Part model, mm, in its own coordinate system. Face numbers are marked on the shaded views. A direction names the side the tool comes from. Round coordinates to 2 decimals unless told otherwise and drop trailing zeros. Loops run counter-clockwise (first coordinate to the right, second up) from the corner with the lowest first, then second, coordinate; pieces in that order, holes last. Notation, with made-up numbers: M 77.25,-36 L 110.25,-36 A18 ccw 110.25,-11 Z; hole C 83.25,11 d3. An arc over 180 degrees is marked long. Answer as CSV lines item,"result". Start each with the question number.
Item 1: Band-saw the part on B-B (z = 0). Give the cut face in (x, y), and give its area (3 significant figures).
Item 2: Mould opens along Z. For the marked faces 1, 2 and 3 say: pulls with the +Z half, pulls with the -Z half, needs draft (parallel to the pull), parting line crosses it, or undercut.
Item 3: Band-saw the part on C-C (y = 20). Give the cut face in (x, z).
Item 4: Which spindle directions (+Z, -Z, +X, -X, +Y, -Y) get a long thin tool onto all of the face, cutting with end or side? Do the marked faces 4, 5, 6, 7 and 8. Say none if no direction does.
Item 5: Wall check: line 1 (Z direction, x = 34.5, y = 11.5); line 2 (Y direction, x = 6.5, z = 44.5). Give the ranges that are in metal, low to high.
Item 6: Band-saw the part on D-D (x = -39). Give the cut face in (y, z).
Item 7: Drop flat-ended pins along their axis: pin 1 Ø4 at (x, z) = (15.5, -36) entering from +Y; pin 2 Ø1.5 at (y, z) = (23.5, 7) entering from +X; pin 3 Ø3 at (y, z) = (25.5, -25) entering from +X. Give the stop position or say it passes through.
Item 8: Band-saw the part on A-A (x = 0). Give the cut face in (y, z), and give its area (3 significant figures).
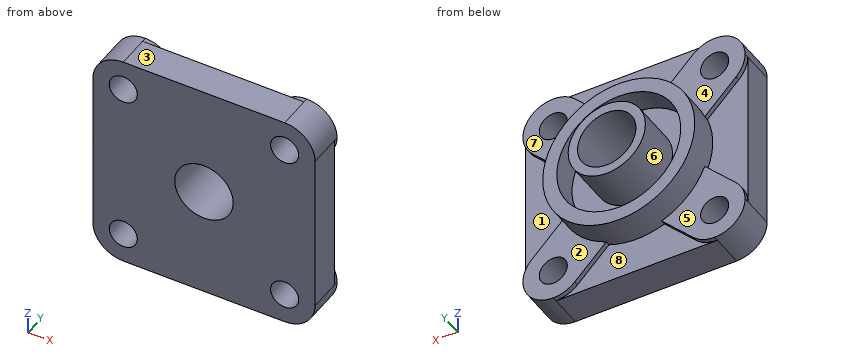
```python
from build123d import *

# Parameters (mm, degrees)
SKETCH1_W           = 95
SKETCH1_H           = 95
BOSS_EXTRUDE1_DEPTH = 14
BOSS_EXTRUDE2_DEPTH = 16
SKETCH4_R           = 32.5
BOSS_EXTRUDE3_DEPTH = 13
SKETCH5_R           = 12.5
CUT_EXTRUDE1_DEPTH  = 73.398204398
SKETCH6_R           = 26.5
SKETCH6_R_2         = 16.5
CUT_EXTRUDE2_DEPTH  = 11
BOSS_EXTRUDE4_START = 35.7
SKETCH7_R           = 16.5
SKETCH7_R_2         = 12.5
BOSS_EXTRUDE4_DEPTH = 35.7
CUT_EXTRUDE3_DEPTH  = 77.072268272
SKETCH9_R           = 6
CUT_EXTRUDE5_DEPTH  = 77.072268272


with BuildPart() as part:
    # Sketch1 → Boss-Extrude1 (new body)
    with BuildSketch(Plane(origin=(0, 0, 0), x_dir=(1, 0, 0), z_dir=(0, 1, 0))):
        Rectangle(SKETCH1_W, SKETCH1_H)
    extrude(amount=BOSS_EXTRUDE1_DEPTH)

    # Sketch2 → Boss-Extrude2 (add)
    with BuildSketch(Plane(origin=(0, 0, 0), x_dir=(1, 0, 0), z_dir=(0, 1, 0))):
        with BuildLine():
            Line((-30.254795425, 11.870019114), (-43.692388155, 25.307611845))
            ThreePointArc((-43.692388155, 25.307611845), (-43.692388155, 43.692388155), (-25.307611845, 43.692388155))
            Line((-25.307611845, 43.692388155), (-11.870019114, 30.254795425))
            ThreePointArc((-11.870019114, 30.254795425), (-22.980970389, 22.980970389), (-30.254795425, 11.870019114))
        make_face()
        with BuildLine():
            Line((11.870019114, 30.254795425), (25.307611845, 43.692388155))
            ThreePointArc((25.307611845, 43.692388155), (43.692388155, 43.692388155), (43.692388155, 25.307611845))
            Line((43.692388155, 25.307611845), (30.254795425, 11.870019114))
            ThreePointArc((30.254795425, 11.870019114), (22.980970389, 22.980970389), (11.870019114, 30.254795425))
        make_face()
        with BuildLine():
            Line((30.254795425, -11.870019114), (43.692388155, -25.307611845))
            ThreePointArc((43.692388155, -25.307611845), (43.692388155, -43.692388155), (25.307611845, -43.692388155))
            Line((25.307611845, -43.692388155), (11.870019114, -30.254795425))
            ThreePointArc((11.870019114, -30.254795425), (22.980970389, -22.980970389), (30.254795425, -11.870019114))
        make_face()
        with BuildLine():
            Line((-11.870019114, -30.254795425), (-25.307611845, -43.692388155))
            ThreePointArc((-25.307611845, -43.692388155), (-43.692388155, -43.692388155), (-43.692388155, -25.307611845))
            Line((-43.692388155, -25.307611845), (-30.254795425, -11.870019114))
            ThreePointArc((-30.254795425, -11.870019114), (-22.980970389, -22.980970389), (-11.870019114, -30.254795425))
        make_face()
    extrude(amount=BOSS_EXTRUDE2_DEPTH)

    # Sketch4 → Boss-Extrude3 (add)
    with BuildSketch(Plane(origin=(0, 14, 0), x_dir=(1, 0, 0), z_dir=(0, 1, 0))):
        with Locations(Location((0, 0, 0), (0, 0, 111.421821522))):
            Circle(SKETCH4_R)
    extrude(amount=BOSS_EXTRUDE3_DEPTH)

    # Sketch5 → Cut-Extrude1 (cut, through all)
    with BuildSketch(Plane(origin=(0, 27, 0), x_dir=(1, 0, 0), z_dir=(0, 1, 0))):
        with Locations(Location((0, 0, 0), (0, 0, 270))):
            Circle(SKETCH5_R)
    extrude(amount=-CUT_EXTRUDE1_DEPTH, mode=Mode.SUBTRACT)

    # Sketch6 → Cut-Extrude2 (cut)
    with BuildSketch(Plane(origin=(0, 27, 0), x_dir=(1, 0, 0), z_dir=(0, 1, 0))):
        with Locations(Location((0, 0, 0), (0, 0, 270))):
            Circle(SKETCH6_R)
        with Locations(Location((0, 0, 0), (0, 0, 270))):
            Circle(SKETCH6_R_2, mode=Mode.SUBTRACT)
    extrude(amount=-CUT_EXTRUDE2_DEPTH, mode=Mode.SUBTRACT)

    # Sketch7 → Boss-Extrude4 (add)
    with BuildSketch(Plane(origin=(0, 0, 0), x_dir=(1, 0, 0), z_dir=(0, 1, 0)).offset(BOSS_EXTRUDE4_START)):
        with Locations(Location((0, 0, 0), (0, 0, 270))):
            Circle(SKETCH7_R)
        with Locations(Location((0, 0, 0), (0, 0, 270))):
            Circle(SKETCH7_R_2, mode=Mode.SUBTRACT)
    extrude(amount=-BOSS_EXTRUDE4_DEPTH)

    # Sketch8 → Cut-Extrude3 (cut, through all)
    with BuildSketch(Plane(origin=(0, 0, 0), x_dir=(1, 0, 0), z_dir=(0, 1, 0))):
        with BuildLine():
            Line((-47.5, -34.5), (-47.5, -47.5))
            Line((-47.5, -47.5), (-34.5, -47.5))
            ThreePointArc((-34.5, -47.5), (-43.692388155, -43.692388155), (-47.5, -34.5))
        make_face()
        with BuildLine():
            Line((-34.5, 47.5), (-47.5, 47.5))
            Line((-47.5, 47.5), (-47.5, 34.5))
            ThreePointArc((-47.5, 34.5), (-43.692388155, 43.692388155), (-34.5, 47.5))
        make_face()
        with BuildLine():
            Line((47.5, 34.5), (47.5, 47.5))
            Line((47.5, 47.5), (34.5, 47.5))
            ThreePointArc((34.5, 47.5), (43.692388155, 43.692388155), (47.5, 34.5))
        make_face()
        with BuildLine():
            Line((34.5, -47.5), (47.5, -47.5))
            Line((47.5, -47.5), (47.5, -34.5))
            ThreePointArc((47.5, -34.5), (43.692388155, -43.692388155), (34.5, -47.5))
        make_face()
    extrude(amount=CUT_EXTRUDE3_DEPTH, mode=Mode.SUBTRACT)

    # Sketch9 → Cut-Extrude5 (cut, through all)
    with BuildSketch(Plane(origin=(0, 0, 0), x_dir=(1, 0, 0), z_dir=(0, 1, 0))):
        with Locations(Location((-34.5, 34.5, 0), (0, 0, 90))):
            Circle(SKETCH9_R)
        with Locations(Location((34.5, 34.5, 0), (0, 0, 90))):
            Circle(SKETCH9_R)
        with Locations(Location((34.5, -34.5, 0), (0, 0, 90))):
            Circle(SKETCH9_R)
        with Locations(Location((-34.5, -34.5, 0), (0, 0, 90))):
            Circle(SKETCH9_R)
    extrude(amount=CUT_EXTRUDE5_DEPTH, mode=Mode.SUBTRACT)


solid = part.part
```
Answer block:
1,outline,"M -47.5,0 L -12.5,0 L -12.5,35.7 L -16.5,35.7 L -16.5,16 L -26.5,16 L -26.5,27 L -32.5,27 L -32.5,14 L -47.5,14 Z; M 12.5,0 L 47.5,0 L 47.5,14 L 32.5,14 L 32.5,27 L 26.5,27 L 26.5,16 L 16.5,16 L 16.5,35.7 L 12.5,35.7 Z"
1,area,"1,350 mm^2"
2,face 1,"undercut"
2,face 2,"needs draft"
2,face 3,"pulls with the +Z half"
3,outline,"C 0,0 d65; C 0,0 d33; hole C 0,0 d53; hole C 0,0 d25"
4,face 4,"+Z, -X, +Y"
4,face 5,"-Z, -X, +Y"
4,face 6,"+Y"
4,face 7,"+Z, +X, +Y"
4,face 8,"-Z, +Y"
5,line 1,"z = -47.5 to -40.5, -28.5 to 28.5, 40.5 to 47.5"
5,line 2,"y = 0 to 14"
6,outline,"M 0,-46.7 L 16,-46.7 L 16,-38.47 L 0,-38.47 Z; M 0,-30.53 L 16,-30.53 L 16,-20.62 L 14,-20.62 L 14,20.62 L 16,20.62 L 16,30.53 L 0,30.53 Z; M 0,38.47 L 16,38.47 L 16,46.7 L 0,46.7 Z"
7,pin 1,"stops at y = 16"
7,pin 2,"stops at x = 31.89"
7,pin 3,"stops at x = 22.45"
8,outline,"M 0,-47.5 L 14,-47.5 L 14,-32.5 L 27,-32.5 L 27,-26.5 L 16,-26.5 L 16,-16.5 L 35.7,-16.5 L 35.7,-12.5 L 0,-12.5 Z; M 0,12.5 L 35.7,12.5 L 35.7,16.5 L 16,16.5 L 16,26.5 L 27,26.5 L 27,32.5 L 14,32.5 L 14,47.5 L 0,47.5 Z"
8,area,"1,350 mm^2"
